Could you check a few things on this drawing? It's one solid part, dimensions in mm from its lowest x, y, z. A direction names the side the tool comes from. Round coordinates to 2 decimals unless told otherwise and drop trailing zeros. Loops run counter-clockwise (first coordinate to the right, second up) from the corner with the lowest first, then second, coordinate; pieces in that order, holes last. Notation, with made-up numbers: (83.25, 85) -> (124.25, 85) arc R23 ccw to (124.25, 96) -> close; hole circle Ø6 at (-22, 9). An arc over 180 degrees is marked (long way). Use one line per item in the form item = value. Start each with the question number.
Item 1: I'm going to push flat-ended pins straight in: pin 1 Ø1 at (x, y) = (23.5, 15) entering from -Z; pin 2 Ø8 at (y, z) = (28, 6) entering from +X; pin 3 Ø18.5 at (x, y) = (47, 32) entering from -Z. Where does each tip first touch, or does it pass through?
Item 2: If we section it at A-A (z = 32.5): Write out the boundary of the cut face in (x, y) (1 decimal).
Item 3: If we section it at C-C (x = 51): Write out the boundary of the cut face in (y, z).
Item 4: If we section it at D-D (z = 7.5): Write out the boundary of the cut face in (x, y), then the cut area to 3 significant figures.
Item 5: For the marked faces 1, 2, 3 and 4, which set-ups out of +Z, -Z, +X, -X, +Y, -Y let a thin tool reach every point of the face, with its end or its side?
Item 6: Thinking about a two-plate mould opening in X: for the marked faces 5, 6 and 7, which applies, released by +X, released by -X, zero draft, split by the parting line, or undercut?
Item 7: If we section it at B-B (y = 24): Write out the boundary of the cut face in (x, z) (1 decimal), then the cut area to 3 significant figures.
Item 8: If I drill on L1, parallel to X at y = 31.5, z = 30 (1 decimal); L2, parallel to Z at x = 27, y = 8; L3, parallel to X at y = 22, z = 3, over which ranges is the centre line in solid material (lowest first)? Write a range as [from, to].
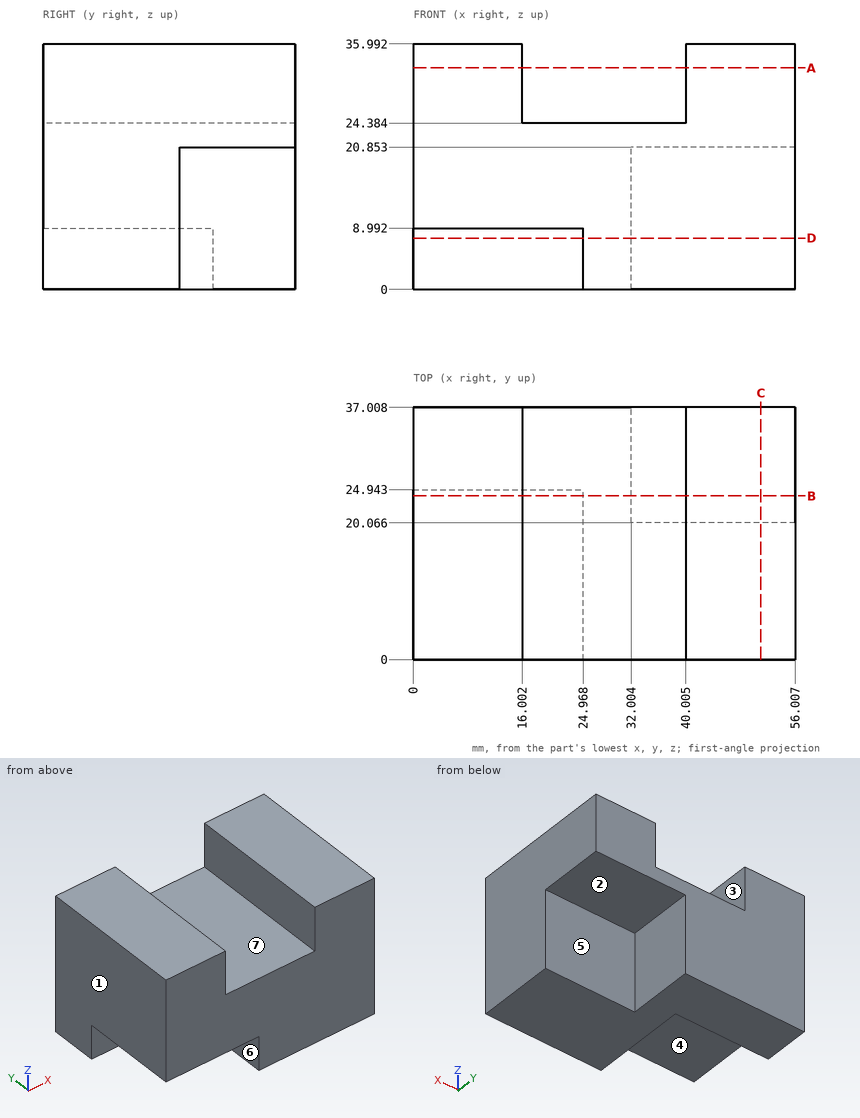
Values found:
q1.pin_1 = 8.99
q1.pin_2 = 32
q1.pin_3 = 20.85
q2.outline = (0, 0) -> (16, 0) -> (16, 37) -> (0, 37) -> close; (40, 0) -> (56, 0) -> (56, 37) -> (40, 37) -> close
q3.outline = (0, 0) -> (20.07, 0) -> (20.07, 20.85) -> (37.01, 20.85) -> (37.01, 35.99) -> (0, 35.99) -> close
q4.outline = (0, 24.94) -> (24.97, 24.94) -> (24.97, 0) -> (56.01, 0) -> (56.01, 20.07) -> (32, 20.07) -> (32, 37.01) -> (0, 37.01) -> close
q4.area = 1,040 mm2
q5.face_1 = +Z, -Z, -X, +Y, -Y
q5.face_2 = -Z, +X, +Y
q5.face_3 = +Z, +Y, -Y
q5.face_4 = -Z, -X, -Y
q6.face_5 = zero draft
q6.face_6 = released by -X
q6.face_7 = undercut
q7.outline = (0, 9) -> (25, 9) -> (25, 0) -> (32, 0) -> (32, 20.9) -> (56, 20.9) -> (56, 36) -> (40, 36) -> (40, 24.4) -> (16, 24.4) -> (16, 36) -> (0, 36) -> close
q7.area = 1,010 mm2
q8.L1 = [0, 16], [40, 56]
q8.L2 = [0, 24.38]
q8.L3 = [24.97, 32]
